```python
from build123d import *

# Parameters (mm, degrees)
F0_R     = 25
F1_DEPTH = 150
F2_W     = 15
F2_H     = 15.545452
F3_DEPTH = 25
F4_W     = 15
F4_H     = 12.647062
F5_DEPTH = 25


with BuildPart() as f1:
    # F0 (on Top) → F1 (new body)
    with BuildSketch(Plane.XY):
        Circle(F0_R)
    extrude(amount=F1_DEPTH)

    # F2 (on face) → F3 (join)
    with BuildSketch(Plane.XY.offset(150)):
        Rectangle(F2_W, F2_H)
    extrude(amount=F3_DEPTH)

    # F4 (on face) → F5 (join)
    with BuildSketch(Plane(origin=(0, 0, 0), x_dir=(1, 0, 0), z_dir=(0, 0, -1))):
        Rectangle(F4_W, F4_H)
    extrude(amount=F5_DEPTH)


solid = f1.part
```
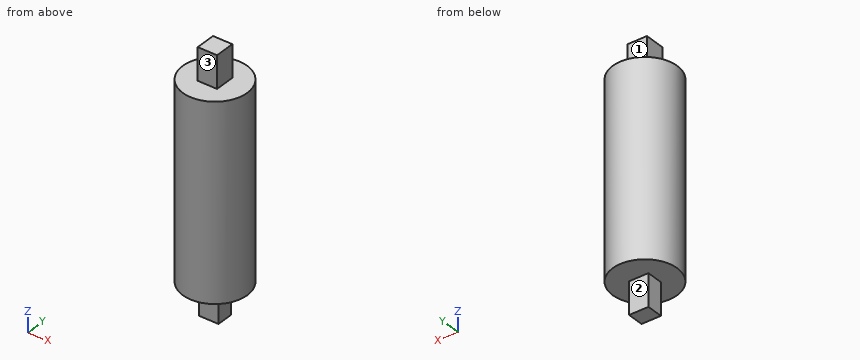
CAD build for the part. Positions are in the model's coordinates, mm. Face numbers are marked on the shaded views. A direction names the side the tool comes from. Round coordinates to 2 decimals unless told otherwise and drop trailing zeros. Loops run counter-clockwise (first coordinate to the right, second up) from the corner with the lowest first, then second, coordinate; pieces in that order, holes last. Notation, with made-up numbers: M -6.75,62 L 31.25,62 A23 ccw 31.25,97 Z; hole C -7,43.5 d3. An arc over 180 degrees is marked long. Use a Markdown table: item, result. Add a question column.
(1) Cut at D-D (y = -20). Give the cut face in (x, z), and give its area (3 significant figures).
(2) Cut at B-B (y = 0). Give the cut face in (x, z), and give its area (3 significant figures).
(3) Cut at A-A (x = 0). Give the cut face in (y, z).
(4) Cut at C-C (z = 62.5). Give the cut face in (x, y).
(5) Which spindle directions (+Z, -Z, +X, -X, +Y, -Y) get a long thin tool onto all of the face, cutting with end or side? Do the marked faces 1, 2 and 3. Say none if no direction does.
(6) Drill centre lines: line 1 (Z direction, x = -15.5, y = -8); line 2 (X direction, y = -13, z = 74.5); line 3 (X direction, y = 0.5, z = 35.5) (3 decimals). Where is each one in solid material? Low to high.
(7) Flat gauge pins, fed straight in: pin 1 (4.5 mm diameter, centred on x = 3, z = -7, fed in from +Y); pin 2 (8 mm diameter, centred on y = -13.5, z = 128.5, fed in from +X); pin 3 (8 mm diameter, centred on y = 0, z = 161, fed in from -X); pin 4 (2 mm diameter, centred on y = -1, z = 39.5, fed in from +X). Where does each tip first touch, or does it go through?
Geometry says:
| question | item | result |
|---|---|---|
| 1 | outline | M -15,0 L 15,0 L 15,150 L -15,150 Z |
| 1 | area | 4,500 mm² |
| 2 | outline | M -25,0 L -7.5,0 L -7.5,-25 L 7.5,-25 L 7.5,0 L 25,0 L 25,150 L 7.5,150 L 7.5,175 L -7.5,175 L -7.5,150 L -25,150 Z |
| 2 | area | 8,250 mm² |
| 3 | outline | M -25,0 L -6.32,0 L -6.32,-25 L 6.32,-25 L 6.32,0 L 25,0 L 25,150 L 7.77,150 L 7.77,175 L -7.77,175 L -7.77,150 L -25,150 Z |
| 4 | outline | C 0,0 d50 |
| 5 | face 1 | +Z, +X, -X, +Y |
| 5 | face 2 | -Z, +X, -X, +Y |
| 5 | face 3 | +Z, +X, -X, -Y |
| 6 | line 1 | z = 0 to 150 |
| 6 | line 2 | x = -21.35 to 21.35 |
| 6 | line 3 | x = -24.995 to 24.995 |
| 7 | pin 1 | stops at y = 6.32 |
| 7 | pin 2 | stops at x = 23.12 |
| 7 | pin 3 | stops at x = -7.5 |
| 7 | pin 4 | stops at x = 25 |
